from build123d import *

# Parameters (mm, degrees)
SKETCH012_R             = 5
PAD004_DEPTH            = 16
SKETCH013_R             = 3.5
POCKET_DEPTH            = 35.001
FILLET_R                = 2
BODY003_PLACEMENT_ANGLE = 0.285111


with BuildPart() as part:
    # Sketch012 → Pad004 (new body)
    with BuildSketch(Plane.XZ):
        with BuildLine():
            Line((33.5, -18), (-33.5, -18))
            Line((-33.5, -18), (-33.5, -12))
            Line((-33.5, -12), (-17, -12))
            Line((-17, -12), (-17, 0))
            ThreePointArc((17, 0), (0, 17), (-17, 0))
            Line((17, 0), (17, -12))
            Line((17, -12), (33.5, -12))
            Line((33.5, -12), (33.5, -18))
        make_face()
        Circle(SKETCH012_R, mode=Mode.SUBTRACT)
    extrude(amount=PAD004_DEPTH)

    # Sketch013 (on Face4 of Pad004) → Pocket (cut, through all)
    with BuildSketch(Plane(origin=(0, 0, -18), x_dir=(1, 0, 0), z_dir=(0, 0, -1))):
        with Locations((-26.5, 8)):
            Circle(SKETCH013_R)
        with Locations((26.5, 8)):
            Circle(SKETCH013_R)
    extrude(amount=-POCKET_DEPTH, mode=Mode.SUBTRACT)

    # Fillet
    fillet_edges = [part.edges().sort_by_distance(p)[0] for p in [
        (0, -16, 17),
        (0, 0, 17),
        (-25.25, 0, -12),
        (-25.25, -16, -12),
        (-33.5, -16, -15),
        (-33.5, 0, -15),
        (25.25, -16, -12),
        (25.25, 0, -12),
        (33.5, 0, -15),
        (33.5, -16, -15),
        (33.5, -8, -12),
    ]]
    fillet(fillet_edges, radius=FILLET_R)


with BuildPart() as part_1:
    # Body003 placement: moved
    add(part.part.moved(Location((-6.054991, -96.20389, 26.128014))).rotate(Axis((-6.054991, -96.20389, 26.128014), (0, 0, 1)), BODY003_PLACEMENT_ANGLE))


solid = part_1.part
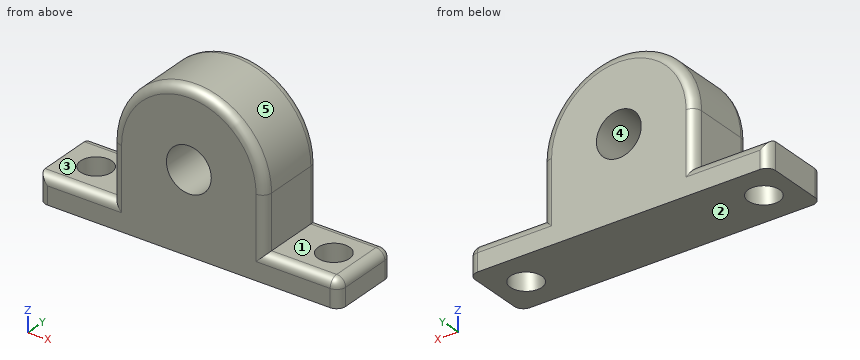
Input: part model. Units: mm. Frame: model coordinates. Face numbers are marked on the shaded views. A direction names the side the tool comes from. Round coordinates to 2 decimals unless told otherwise and drop trailing zeros. Order: outer loops, then holes, each group sorted by start corner. A loop starts at its lowest first (then second) coordinate and runs counter-clockwise, first axis right, second up.
1. Pin query (flat end, axial travel): P1, Ø1, axis at x = 4, z = 14.5, coming from the +Y side; P2, Ø9.5, axis at x = -29.5, y = -104.5, coming from the +Z side; P3, Ø1, axis at y = -103.5, z = 39, coming from the +X side. Return the tip coordinate at first contact, or that it passes through.
The answers:
P1: stops at y = -96.15
P2: stops at z = 14.13
P3: stops at x = 5.64
2. Cut plane B-B, the plane y = -106. State how many separate pieces and enclosed holes the cut face has, then the cut area to 3 significant figures.
The answers:
separate pieces: 3
enclosed holes: 1
area: 1,110 mm2
3. Cut plane A-A, the plane z = 22. Output: boundary loops of the cut face in (x, y).
The answers:
outline: (-23.04, -98.29) - (-22.99, -110.29) arc R2 ccw to (-20.98, -112.28) - (-8.8, -112.22) - (-8.88, -96.22) - (-21.05, -96.28) arc R2 ccw to start; (-3.23, -96.19) - (-3.15, -112.19) - (9.02, -112.13) arc R2 ccw to (11.01, -110.12) - (10.95, -98.12) arc R2 ccw to (8.94, -96.13) - close
4. Material intervals for line 1 (X direction, y = -103.5, z = 13.5); line 2 (Y direction, x = 7, z = 30); line 3 (Z direction, x = -35.5, y = -107.25), sorted ascending.
The answers:
line 1: x = -39.52 to -35.91, -29.12 to 17.03, 23.94 to 26.94
line 2: y = -112.14 to -96.14
line 3: z = 8.13 to 14.13
5. Cut plane C-C, the plane z = 13. Output: boundary loops of the cut face in (x, y) (1 decimal).
The answers:
outline: (-39.5, -110.4) arc R2 ccw to (-38.3, -112.2) - (-21.8, -112.1) arc R2 ccw to (-21, -112.3) - (9, -112.1) arc R2 ccw to (9.9, -111.9) - (25.5, -111.8) arc R1.8 ccw to (27.3, -110) - (27.3, -98) arc R1.8 ccw to (25.4, -96.2) - (9.8, -96.3) arc R2 ccw to (8.9, -96.1) - (-21.1, -96.3) arc R2 ccw to (-21.9, -96.5) - (-38.4, -96.6) arc R2 ccw to (-39.5, -98.4) - close; hole circle Ø7 at (-32.5, -104.3); hole circle Ø7 at (20.5, -104.1)
6. Mould query, pull axis X, two halves, no side actions, for the marked faces 3, 4 and 5. Classes: released by +X, released by -X, zero draft, split by the parting line, or undercut.
The answers:
face 3: zero draft
face 4: undercut
face 5: split by the parting line
7. Set-up query: the marked faces 1 and 2. Return all of +Z, -Z, +X, -X, +Y, -Y with unobstructed straight access to the full face (end or side cutting, diameter ignored); none if empty.
The answers:
face 1: +Z, +X, +Y, -Y
face 2: -Z, +X, -X, +Y, -Y
